```python
from build123d import *

# Parameters (mm, degrees)
EXTRUDE_1_DEPTH        = 1
SM_EDGE_FLANGE_1_DEPTH = 1410


# Sheet-metal steps are written as plain solids
with BuildPart() as part:
    # Sketch 1 → Бобышка-Вытянуть1 (new body)
    with BuildSketch(Plane(origin=(0, 0, 0), x_dir=(1, 0, 0), z_dir=(0, 1, 0))):
        Polygon((0, 0), (20, -20), (1390, -20), (1410, 0), align=None)
    extrude(amount=EXTRUDE_1_DEPTH)

    # Ребро-кромка1 section (across the edge) → Ребро-кромка1 (add)
    with BuildSketch(Plane(origin=(1410, 1, -2.182617002), x_dir=(0, -0.08715574274765482, 0.9961946980917459), z_dir=(-1, 0, 0))):
        with BuildLine():
            Line((-1, 2.182617002), (-1, 8.908691499))
            Line((-1, 8.908691499), (0, 8.908691499))
            Line((0, 8.908691499), (0, 2.182617002))
            ThreePointArc((0, 2.182617002), (0.648819585, 0.708062329), (2.174311485, 0.190227606))
            Line((2.174311485, 0.190227606), (2.261467228, -0.805967092))
            ThreePointArc((2.261467228, -0.805967092), (-0.026770623, -0.029215008), (-1, 2.182617002))
        make_face()
    extrude(amount=SM_EDGE_FLANGE_1_DEPTH)


solid = part.part
```
Geometry check sheet. Reference: the model listing, model coordinates, mm. Round coordinates to 2 decimals unless told otherwise and drop trailing zeros. Order: outer loops, then holes, each group sorted by start corner. A loop starts at its lowest first (then second) coordinate and runs counter-clockwise, first axis right, second up. Notation, with made-up numbers: (80.25, 57.5) -> (101.25, 57.5) arc R34 cw to (101.25, 95.5) -> close; hole circle Ø11 at (84.5, 19.5). An arc over 180 degrees is marked (long way). Return JSON: item names as keys, results as strings. Group by question number.
Q1. Section check A-A, the plane x = 386. Record the boundary of the cut face in (y, z), plus the area to 3 significant figures.
Q2. Section check C-C, the plane y = 5. Record the boundary of the cut face in (x, z).
Q3. Gauge pin test, flat ends, axial feed: pin 1 (8 mm diameter, centred on x = 1194, z = 13, fed in from +Y); pin 2 (1 mm diameter, centred on x = 571, y = 4, fed in from +Z). Record the tip position at first contact, or that the pin passes through.
Q4. Material ranges on probe 1 along Y at (x, z) = (323.5, -0.75); probe 2 along Z at (x, y) = (1289, 0.5); probe 3 along Y at (x, z) = (1199.5, 16.5), recorded low to high. Write a range as from..to.
Q5. Section check B-B, the plane z = 3.5. Record the boundary of the cut face in (x, y).
Numbers:
{
 "1": {"outline": "(0, 0) arc R3 ccw to (3.26, -2.99) -> (9.96, -2.4) -> (9.87, -1.41) -> (3.17, -1.99) arc R2 cw to (1, 0) -> (1, 20) -> (0, 20) -> close", "area": "30.9 mm^2"},
 "2": {"outline": "(0, -2.84) -> (1410, -2.84) -> (1410, -1.83) -> (0, -1.83) -> close"},
 "3": {"pin 1": "y = 1", "pin 2": "z = -1.88"},
 "4": {"probe 1": "0.1..1.15", "probe 2": "-1.66..20", "probe 3": "0..1"},
 "5": {"outline": "(3.5, 0) -> (1406.5, 0) -> (1406.5, 1) -> (3.5, 1) -> close"}
}
